Input: part model. Units: mm. Frame: model coordinates. Give positions to 0.01 mm unless a question says otherwise; leave off trailing zeros. Loops run counter-clockwise (first coordinate to the right, second up) from the corner with the lowest first, then second, coordinate; pieces in that order, holes last. Notation, with made-up numbers: M 25,76.5 L 63,76.5 A22 cw 63,110.5 Z; hole C 9,-9.75 d8. An arc over 180 degrees is marked long. Answer as a JSON object with one key per item and string values. Group by question number.
1) Section query C-C on z = 147. Return loops of the section in (x, y).
2) First-contact query: P1, Ø6, axis at y = -3, z = 79.5, coming from the -X side; P2, Ø1, axis at x = 3, z = 252.5, coming from the -Y side; P3, Ø2, axis at x = -0.5, y = -2, coming from the +Z side; P4, Ø5, axis at x = 1, y = -1, coming from the +Z side. Flat tips, straight axial feed; report the tip coordinate or a pass-through.
3) Ray query, L1, parallel to X at y = 0, z = 84.5; L2, parallel to Z at x = 0.75, y = 0; L3, parallel to Z at x = 4.25, y = 1.5. Return the intervals inside material, ascending.
4) Section query A-A on x = 0. Return loops of the section in (y, z).
from build123d import *

# Parameters (mm, degrees)
F0_R     = 3.8
F1_DEPTH = 305


with BuildPart() as f1:
    # F0 (on Top) → F1 (new body)
    with BuildSketch(Plane.XY):
        Circle(F0_R)
    extrude(amount=F1_DEPTH)

    # F3 (on offset) → F4 (revolve)
    with BuildSketch(Plane.XY.offset(308)):
        with BuildLine():
            Line((0, -5), (0, 5))
            ThreePointArc((0, 5), (-5, 0), (0, -5))
        make_face()
    revolve(axis=Axis((0, 0, 308), (0, -1, 0)))

    # F6 (on offset) → F7 (revolve)
    with BuildSketch(Plane(origin=(0, 0, -3), x_dir=(1, 0, 0), z_dir=(0, 0, -1))):
        with BuildLine():
            Line((0, -5), (0, 5))
            ThreePointArc((0, 5), (-5, 0), (0, -5))
        make_face()
    revolve(axis=Axis((0, 0, -3), (0, 1, 0)))


solid = f1.part
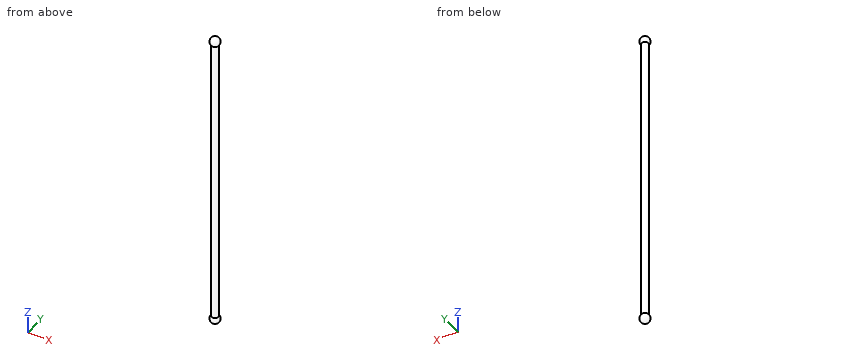
Output:
{
 "1": {"outline": "C 0,0 d7.6"},
 "2": {"P1": "stops at x = -3.8", "P2": "stops at y = -2.86", "P3": "stops at z = 312.89", "P4": "stops at z = 313"},
 "3": {"L1": "x = -3.8 to 3.8", "L2": "z = -7.94 to 312.94", "L3": "z = -5.17 to -0.83, 305.83 to 310.17"},
 "4": {"outline": "M -3.8,0.25 A5 ccw long 3.8,0.25 L 3.8,304.75 A5 ccw long -3.8,304.75 Z"}
}
